The model under review builds one solid part; all positions refer to its coordinate system, in mm. Face numbers are marked on the shaded views. A direction names the side the tool comes from. Round coordinates to 2 decimals unless told otherwise and drop trailing zeros. Order: outer loops, then holes, each group sorted by start corner. A loop starts at its lowest first (then second) coordinate and runs counter-clockwise, first axis right, second up.
1) Consider section B-B (y = 0). Give the boundary of the cut face in (x, z).
2) To check wall thickness, follow L1, parallel to Z at x = 4.75, y = -0.75; L2, parallel to Z at x = 1.25, y = -1.25; L3, parallel to Y at x = -0.5, z = 2.75. State the ranges of each line that lie inside material, in increasing order.
3) Consider section D-D (x = -2). Give the boundary of the cut face in (y, z).
4) Machinability: for the marked faces 1, 2 and 3, which of the approach directions +Z, -Z, +X, -X, +Y, -Y give a long, thin tool a straight path to every point of the face, cutting with its end or side? Answer none if there is none.
5) Consider section A-A (x = 4.5). Give the boundary of the cut face in (y, z), then the cut area to 3 significant figures.
6) Mouldability with a two-part tool opening along Z and no side actions: class the marked faces 4, 5, 6 and 7 as pulls with the +Z half, pulls with the -Z half, needs draft (parallel to the pull), parting line crosses it, or undercut.
7) Clearance check with flat-ended pins moving along their axes: P1, Ø2.5, axis at x = 0, z = 5, coming from the -Y side; P2, Ø1.7, axis at x = 3.5, z = 1, coming from the +Y side; P3, Ø1.1, axis at x = 4, z = 8, coming from the +Y side; P4, Ø4, axis at x = 5, z = 1.5, coming from the -Y side. State where each tip first meets the part, or that it passes through.
8) Consider section C-C (y = -2.75). Give the boundary of the cut face in (x, z).
Autodesk Inventor part; units mm, degrees
ref_plane "YZ Plane" through (0, 0, 0) normal (1, 0, 0) x (0, 1, 0)
ref_plane "XZ Plane" through (0, 0, 0) normal (0, 1, 0) x (-1, 0, 0)
ref_plane "XY Plane" through (0, 0, 0) normal (0, 0, 1) x (1, 0, 0)
sketch "Sketch1" plane through (0, 0, 0) normal (0, 0, 1) x (1, 0, 0)
  line L0 (-0.7045, 1.4865) -> (6.0955, 1.4865)
  line L1 (6.0955, 1.4865) -> (6.0955, -2.5135)
  line L2 (6.0955, -2.5135) -> (-0.7045, -2.5135)
  line L3 (-0.7045, -2.5135) -> (-0.7045, 1.4865)
  line L4 (0.9955, 1.4865) -> (0.9955, 0.4865)
  line L5 (0.9955, 0.4865) -> (5.4766, 0.4865)
  line L6 (5.4766, 0.4865) -> (6.0955, 0.2015)
  line L7 (-0.7045, -1.0135) -> (-2.2782, -1.0135)
  line L8 (-2.2782, -1.0135) -> (-2.7045, -1.3759)
  line L9 (-2.7045, -1.3759) -> (-2.7045, -2.5135)
  line L10 (-2.7045, -2.5135) -> (-0.7045, -2.5135)
  point P0 (0, 0)
  dimension "d0" = 6.8
  dimension "d1" = 4
  dimension "d2" = 1.7
  dimension "d3" = 1
  dimension "d4" = 8.8
  dimension "d5" = 1.5
extrude "Extrusion1" add sketch "Sketch1" along normal blind 9.8 contours L0 L4 L5 L6 L1 L2 L3 | L3 L10 L9 L8 L7
sketch "Sketch2" plane through (0.9955, 0.4865, 0) normal (0, 1, 0) x (1, 0, 0)
  line L0 (0, 0) -> (0, -9.8)
  line L1 (4.4812, -9.8) -> (0, -9.8)
  line L2 (6, -0.4) -> (0, -0.4)
  line L3 (0, -0.4) -> (0, -9.4)
  line L4 (0, -9.4) -> (6, -9.4)
  line L5 (6, -9.4) -> (6, -0.4)
  point P0 (-0.9955, 0)
  dimension "d8" = 9
  dimension "d9" = 0.4
  dimension "d10" = 6
extrude "Extrusion2" cut sketch "Sketch2" against normal blind 2
sketch "Sketch3" plane through (0.9955, -1.5135, 0) normal (0, 1, 0) x (1, 0, 0)
  line L0 (0, -9.4) -> (0, -0.4)
  line L1 (0, -6.5) -> (5.6296, -6.5)
  line L2 (5.6296, -6.5) -> (5.6296, -7.3)
  line L3 (5.6296, -7.3) -> (0, -7.3)
  line L4 (0, -7.3) -> (0, -6.5)
  line L5 (0, -2.5) -> (5.6296, -2.5)
  line L6 (5.6296, -2.5) -> (5.6296, -3.3)
  line L7 (5.6296, -3.3) -> (0, -3.3)
  line L8 (0, -3.3) -> (0, -2.5)
  line L9 (4.4812, -9.8) -> (0, -9.8)
  point P0 (-0.9955, 0)
  dimension "d13" = 0.8
  dimension "d14" = 0.8
  dimension "d15" = 3.2
  dimension "d16" = 3.3
extrude "Extrusion3" cut sketch "Sketch3" against normal blind 0.6
sketch "Sketch6" plane through (6.0955, -2.5135, 0) normal (1, 0, 0) x (0, 0, -1)
  line L0 (-3.3, 1) -> (-6.5, 1)
  line L1 (-7.3, 1) -> (-9.4, 1)
  line L2 (-9.8, 0) -> (-9.8, 2.715)
  line L3 (-0.4, 1) -> (-2.5, 1)
  circle A0 centre (-7.6, 2) radius 0.3
  circle A1 centre (-5.6, 2) radius 0.3
  circle A2 centre (-3.6, 2) radius 0.3
  circle A3 centre (-1.6, 2) radius 0.3
  point P0 (0, 2.5135)
  dimension "d21" = 2.2
  dimension "d22" = 2
  dimension "d23" = 2
  dimension "d24" = 2
  dimension "d25" = 1
  dimension "d26" = 1
  dimension "d27" = 1
  dimension "d28" = 1
  dimension "d29" = 0.6
  dimension "d30" = 0.6
  dimension "d31" = 0.6
  dimension "d32" = 0.6
extrude "Extrusion4" add sketch "Sketch6" against normal blind 7
sketch "Sketch8" plane through (-2.2782, -1.0135, 0) normal (0, 1, 0) x (1, 0, 0)
  line L0 (1.5737, 0) -> (0, 0)
  line L1 (1.5737, 0) -> (1.5737, -9.8)
  line L2 (1.5737, -9.8) -> (-2.262, -9.8)
  line L3 (-2.262, -9.8) -> (-2.2372, 0)
  line L4 (-2.2372, 0) -> (1.2362, 0)
  line L5 (-0.8777, -0.4503) -> (1.2362, 0)
  line L6 (-0.8777, -0.4503) -> (-0.8777, -0.7872)
  line L7 (-0.8777, -0.7872) -> (1.5737, -1.307)
  line L8 (1.5737, -1.307) -> (1.5737, -1.9292)
  line L9 (1.5737, -1.9292) -> (-0.9327, -2.463)
  line L10 (-0.9327, -2.463) -> (-0.9327, -2.783)
  line L11 (-0.9327, -2.783) -> (1.5737, -3.3145)
  line L12 (1.5737, -3.3145) -> (1.5737, -3.9081)
  line L13 (1.5737, -3.9081) -> (-1.0204, -4.4607)
  line L14 (-1.0204, -4.4607) -> (-1.0204, -4.7289)
  line L15 (-1.0204, -4.7289) -> (1.5737, -5.3179)
  line L16 (1.5737, -5.3179) -> (1.5737, -5.906)
  line L17 (1.5737, -5.906) -> (-0.9385, -6.4411)
  line L18 (-0.9385, -6.4411) -> (-0.9385, -6.767)
  line L19 (-0.9385, -6.767) -> (1.5737, -7.3035)
  line L20 (1.5737, -7.3035) -> (1.5737, -7.9182)
  line L21 (1.5737, -7.9182) -> (-1.0783, -8.4831)
  line L22 (-1.0783, -8.4831) -> (-1.0783, -9.2337)
  line L23 (-1.0783, -9.2337) -> (1.5737, -9.8)
  point P0 (2.2782, 0)
extrude "Extrusion5" cut sketch "Sketch8" against normal through all contours L5 L6 L7 L1 L9 L10 L11 L13 L14 L15 L17 L18 L19 L21 L22 L23 L2 L3 L4 L0
sketch "Sketch9" plane through (6.0955, -2.5135, 0) normal (0, -1, 0) x (1, 0, 0)
  line L0 (-6.8, 5.906) -> (-6.8, 5.3179)
  line L1 (-6.8, 3.9081) -> (-6.8, 3.3145)
  line L2 (-6.8, 1.9292) -> (-6.8, 1.307)
  line L3 (-6.8, 7.9182) -> (-6.8, 7.3035)
  circle A0 centre (-6.8, 1.6113) radius 0.3
  circle A1 centre (-6.8, 7.6108) radius 0.3
  circle A2 centre (-6.8, 5.612) radius 0.3
  circle A3 centre (-6.8, 3.6113) radius 0.3
  point P0 (-6.0955, 0)
  dimension "d54" = 0.6
  dimension "d56" = 0.6
  dimension "d57" = 0.6
  dimension "d58" = 0.6
  dimension "d59" = 2
extrude "Extrusion6" add sketch "Sketch9" along normal blind 3.2 and the other way blind 2
properties part number "2mmWireBoardConn"
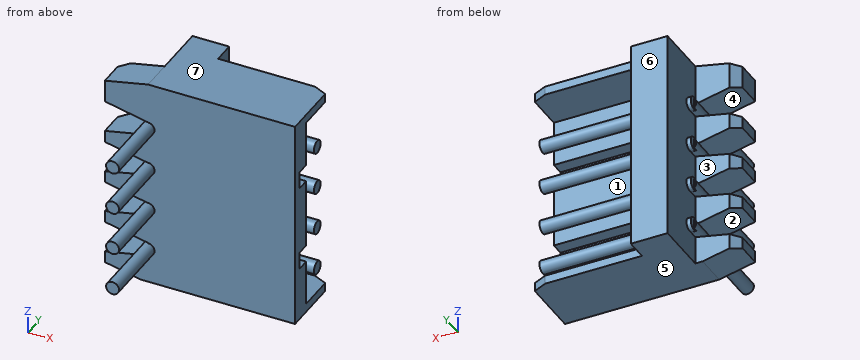
Answer below:
1. outline: (-0.7, 0) - (6.1, 0) - (6.1, 0.4) - (1, 0.4) - (1, 9.4) - (6.1, 9.4) - (6.1, 9.8) - (-0.7, 9.8) - close
2. L1: z = 0 to 0.4, 1.42 to 1.78, 3.42 to 3.78, 5.42 to 5.78, 7.42 to 7.78, 9.4 to 9.8
2. L2: z = 0 to 0.4, 9.4 to 9.8
2. L3: y = -2.51 to 1.49
3. outline: (-2.51, 0.2) - (-1.01, 0.2) - (-1.01, 1.03) - (-2.51, 1.03) - close; (-2.51, 2.21) - (-1.01, 2.21) - (-1.01, 3.04) - (-2.51, 3.04) - close; (-2.51, 4.18) - (-1.01, 4.18) - (-1.01, 5.02) - (-2.51, 5.02) - close; (-2.51, 6.18) - (-1.01, 6.18) - (-1.01, 7.03) - (-2.51, 7.03) - close; (-2.51, 8.19) - (-1.01, 8.19) - (-1.01, 9.52) - (-2.51, 9.52) - close
4. face 1: +X
4. face 2: -X, +Y, -Y
4. face 3: -X, +Y
5. outline: (-2.51, 0) - (0.49, 0) - (0.49, 0.4) - (-1.51, 0.4) - (-1.51, 2.5) - (-2.11, 2.5) - (-2.11, 3.3) - (-1.51, 3.3) - (-1.51, 6.5) - (-2.11, 6.5) - (-2.11, 7.3) - (-1.51, 7.3) - (-1.51, 9.4) - (0.49, 9.4) - (0.49, 9.8) - (-2.51, 9.8) - close; circle Ø0.6 at (-0.51, 1.6); circle Ø0.6 at (-0.51, 3.6); circle Ø0.6 at (-0.51, 5.6); circle Ø0.6 at (-0.51, 7.6)
5. area: 11.6 mm2
6. face 4: undercut
6. face 5: pulls with the -Z half
6. face 6: needs draft
6. face 7: pulls with the +Z half
7. P1: stops at y = -5.71
7. P2: stops at y = 0.49
7. P3: stops at y = -0.21
7. P4: stops at y = -2.51
8. outline: circle Ø0.6 at (-0.7, 1.61); circle Ø0.6 at (-0.7, 3.61); circle Ø0.6 at (-0.7, 5.61); circle Ø0.6 at (-0.7, 7.61)
